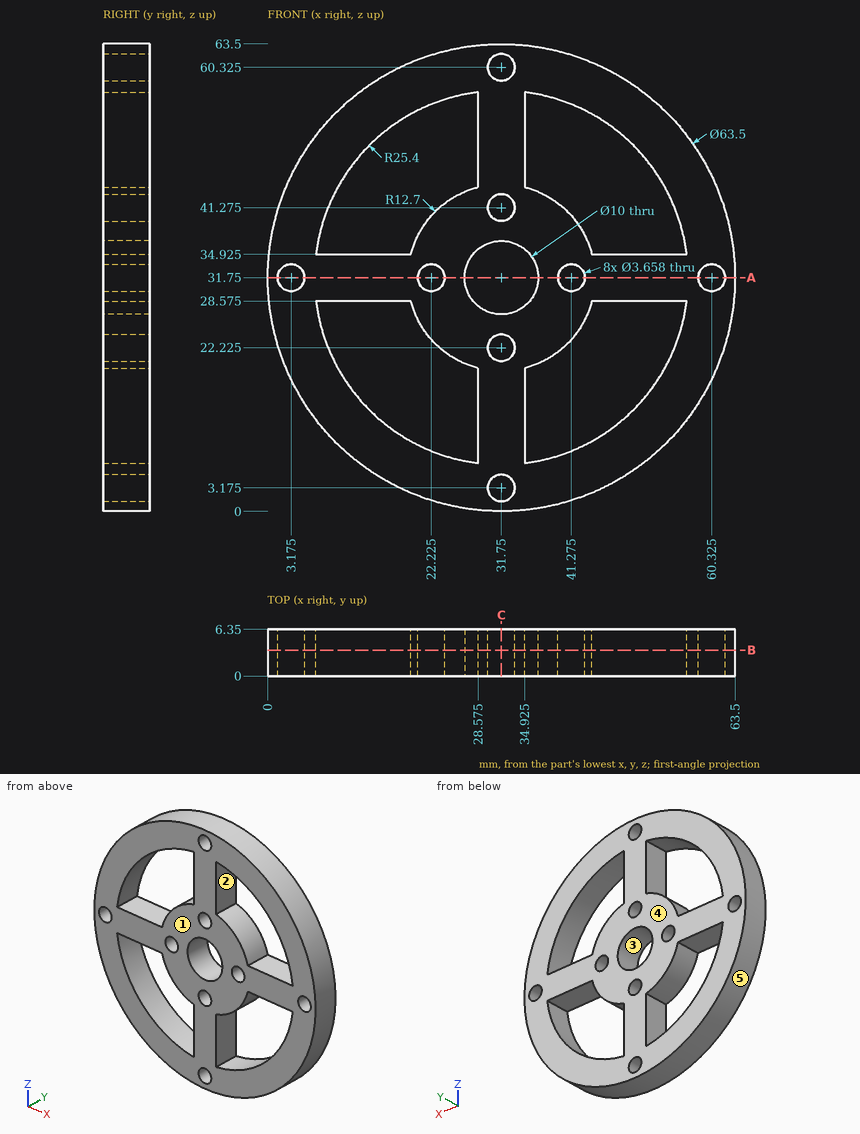
Geometry check sheet. Reference: drawing and pictorial views, mm from the part's lowest x, y, z. A direction names the side the tool comes from. Coordinates: 2 decimals unless noted, no trailing zeros. Loops run counter-clockwise (first coordinate to the right, second up) from the corner with the lowest first, then second, coordinate; pieces in that order, holes last.
1) Sectioned sample at A-A (z = 31.75). Record the boundary of the cut face in (x, y), and give its area (3 significant figures).
2) Release check for a two-part mould opening along X. For the marked faces 3, 4 and 5 record: released by +X, released by -X, zero draft, split by the parting line, or undercut.
3) Material ranges on probe 1 along X at (y, z) = (3.5, 32); probe 2 along X at (y, z) = (3.25, 12.5) (1 decimal); probe 3 along X at (y, z) = (1, 18) (1 decimal), recorded low to high.
4) Access from +Z, -Z, +X, -X, +Y, -Y to the whole of each face (thin tool, end or side, straight path). Record for the marked faces 1 and 2.
5) Gauge pin test, flat ends, axial feed: pin 1 (1.5 mm diameter, centred on x = 24.5, z = 55.5, fed in from +Y); pin 2 (1.9 mm diameter, centred on y = 2, z = 49.5, fed in from +X); pin 3 (2 mm diameter, centred on x = 31.75, z = 41.275, fed in from +Y); pin 4 (3 mm diameter, centred on x = 14, y = 1.5, fed in from +Z). Record the tip position at first contact, or that the pin passes through.
6) Sectioned sample at C-C (x = 31.75). Record the boundary of the cut face in (y, z).
7) Sectioned sample at B-B (y = 3.5). Count the separate pieces of the cut face and the enclosed holes in it, and give its area (3 significant figures).
Check sheet entries:
1. outline: (0, 0) - (1.35, 0) - (1.35, 6.35) - (0, 6.35) - close; (5, 0) - (20.4, 0) - (20.4, 6.35) - (5, 6.35) - close; (24.05, 0) - (26.75, 0) - (26.75, 6.35) - (24.05, 6.35) - close; (36.75, 0) - (39.45, 0) - (39.45, 6.35) - (36.75, 6.35) - close; (43.1, 0) - (58.5, 0) - (58.5, 6.35) - (43.1, 6.35) - close; (62.15, 0) - (63.5, 0) - (63.5, 6.35) - (62.15, 6.35) - close
1. area: 247 mm2
2. face 3: undercut
2. face 4: zero draft
2. face 5: split by the parting line
3. probe 1: x = 0 to 1.36, 4.99 to 20.41, 24.04 to 26.76, 36.74 to 39.46, 43.09 to 58.51, 62.14 to 63.5
3. probe 2: x = 6.5 to 15.2, 28.6 to 34.9, 48.3 to 57
3. probe 3: x = 3.1 to 10.4, 28.6 to 34.9, 53.1 to 60.4
4. face 1: +Z, -Z, +X, -X, -Y
4. face 2: +Y, -Y
5. pin 1: stops at y = 6.35
5. pin 2: stops at x = 58.69
5. pin 3: passes through
5. pin 4: stops at z = 59.03
6. outline: (0, 0) - (6.35, 0) - (6.35, 1.35) - (0, 1.35) - close; (0, 5) - (6.35, 5) - (6.35, 20.4) - (0, 20.4) - close; (0, 24.05) - (6.35, 24.05) - (6.35, 26.75) - (0, 26.75) - close; (0, 36.75) - (6.35, 36.75) - (6.35, 39.45) - (0, 39.45) - close; (0, 43.1) - (6.35, 43.1) - (6.35, 58.5) - (0, 58.5) - close; (0, 62.15) - (6.35, 62.15) - (6.35, 63.5) - (0, 63.5) - close
7. separate pieces: 1
7. enclosed holes: 13
7. area: 1,810 mm2
